Autodesk Inventor part; units mm, degrees
ref_plane "YZ Plane" through (0, 0, 0) normal (1, 0, 0) x (0, 1, 0)
ref_plane "XZ Plane" through (0, 0, 0) normal (0, 1, 0) x (-1, 0, 0)
ref_plane "XY Plane" through (0, 0, 0) normal (0, 0, 1) x (1, 0, 0)
sketch "Sketch1" plane through (0, 0, 0) normal (0, 0, 1) x (1, 0, 0)
  line L0 (-25, -25) -> (25, -25)
  line L1 (25, -25) -> (25, 25)
  line L2 (25, 25) -> (-25, 25)
  line L3 (-25, 25) -> (-25, -25)
  line L4 (-25, -25) -> (25, 25) construction
  line L5 (25, -25) -> (-25, 25) construction
  line L6 (-25, 0) -> (25, 0) construction
  circle A0 centre (-12, 0) radius 1.75
  line L7 (0, 25) -> (0, -25) construction
  circle A1 centre (12, 0) radius 1.75
  line L8 (-25, 25) -> (25, 25)
  line L9 (25, 25) -> (25, 50)
  line L10 (25, 50) -> (-25, 50)
  line L11 (-25, 50) -> (-25, 25)
  line L12 (-20, 45) -> (-17, 45)
  line L13 (-17, 45) -> (-17, 39)
  line L14 (-17, 39) -> (-20, 39)
  line L15 (-20, 39) -> (-20, 45)
  line L16 (20, 45) -> (17, 45)
  line L17 (17, 45) -> (17, 39)
  line L18 (17, 39) -> (20, 39)
  line L19 (20, 39) -> (20, 45)
  point P0 (0, 0)
  dimension "d0" = 50
  dimension "d1" = 50
  dimension "d14" = 3.5
  dimension "d15" = 24
  dimension "d16" = 25
  dimension "d17" = 5
  dimension "d18" = 6
  dimension "d19" = 3
  dimension "d20" = 17
extrude "Extrusion1" add sketch "Sketch1" along normal blind 5
sketch "Sketch2" plane through (-25, -25, 0) normal (0, -1, 0) x (1, 0, 0)
  line L0 (0, 0) -> (50, 0)
  line L1 (0, 5) -> (50, 5)
  line L2 (0, 0) -> (0, 5)
  arc A0 (17.3396, 24.4279) -> (32.6604, 24.4279) centre (25, 18) ccw
  circle A1 centre (25, 18) radius 17 construction
  line L3 (25, 18) -> (25, 0) construction
  line L4 (0, 5) -> (0, 18)
  arc A2 (50, 18) -> (0, 18) centre (25, 18) ccw
  line L5 (50, 18) -> (50, 5)
  line L6 (25, 18) -> (25, 43) construction
  line L7 (17.3396, 24.4279) -> (20.3369, 28)
  line L8 (25, 33.5572) -> (29.6631, 28)
  line L9 (50, 0) -> (50, 5)
  line L10 (20.3369, 28) -> (29.6631, 28)
  arc A3 (32.6604, 24.4279) -> (25, 28) centre (25, 18) ccw
  arc A4 (25, 28) -> (17.3396, 24.4279) centre (25, 18) ccw
  arc A5 (25, 28) -> (17.3396, 24.4279) centre (25, 18) ccw
  arc A6 (32.6604, 24.4279) -> (25, 28) centre (25, 18) ccw
  line L11 (29.6631, 28) -> (32.6604, 24.4279)
  line L12 (20.3369, 28) -> (25, 33.5572)
  dimension "d4" = 20
  dimension "d5" = 34
  dimension "d6" = 18
  dimension "d24" = 80
extrude "Extrusion2" add sketch "Sketch2" against normal blind 8 contours L4 A2 L5 L1 | A4 A3 A0 | L7 L10 A4 | A3 L10 L11 | L12 L8 L10
sketch "Sketch3" plane through (0, 0, 0) normal (1, 0, 0) x (0, 1, 0)
  line L0 (-17, 28) -> (-25, 28)
  line L1 (-17, 8) -> (-17, 5)
  line L2 (-17, 5) -> (50, 5)
  line L3 (50, 0) -> (-25, 0)
  line L4 (-25, 0) -> (-25, 8)
  line L5 (-25, 43) -> (-17, 43)
  line L6 (-17, 43) -> (-17, 28)
  line L7 (-25, 8) -> (-17, 8)
  line L8 (-25, 28) -> (-25, 43)
  line L9 (-25, 8) -> (-25, 28)
  line L10 (-25, 18) -> (31, 18)
  line L11 (9, 29) -> (31, 35)
  line L12 (31, 18) -> (31, 35)
  line L13 (50, 5) -> (50, 0)
  line L14 (9, 29) -> (-17, 28)
  line L15 (31, 18) -> (56.5287, 18)
  line L16 (56.5287, 18) -> (56.5287, 35)
  line L17 (56.5287, 35) -> (31, 35)
  line L18 (31, 35) -> (31, 18)
  point P0 (0, 0)
  dimension "d9" = 26
  dimension "d10" = 22
  dimension "d11" = 11
  dimension "d12" = 17
revolve "Revolution1" cut sketch "Sketch3" angle 360 about axis through (0, -25, 18) along (0, 1, 0) contours L14 L11 L12 L10 L9 L0 | L17 L16 L15 L12
sketch "Sketch4" plane through (-25, -25, 0) normal (-1, 0, 0) x (0, 0, 1)
  line L0 (5, 8) -> (18, 8)
  line L1 (5, 75) -> (5, 8)
  line L2 (18, 8) -> (5, 58)
  point P0 (0, 25)
  dimension "d21" = 50
extrude "Extrusion3" add sketch "Sketch4" against normal blind 4
mirror "Mirror1" about plane through (0, 0, 0) normal (1, 0, 0) of "Extrusion3"
sketch "Szkic5" plane through (-25, -25, 0) normal (0, -1, 0) x (1, 0, 0)
  circle A0 centre (25, 18) radius 10
  line L0 (20.3369, 28) -> (29.6631, 28)
  line L1 (17.3396, 24.4279) -> (20.3369, 28)
  line L2 (29.6631, 28) -> (32.6604, 24.4279)
  point P0 (25, 0)
extrude "Wyciągnięcie proste4" cut sketch "Szkic5" against normal up to next contours A0 L0 L2 | L1 L0 A0
properties part number "proxxon_mount"
Build history of the part. All positions in model axes, mm. A direction names the side the tool comes from. Give positions to 0.01 mm unless a question says otherwise; leave off trailing zeros. Loops run counter-clockwise (first coordinate to the right, second up) from the corner with the lowest first, then second, coordinate; pieces in that order, holes last. Notation, with made-up numbers: (6.5, 40) - (55.5, 40) arc R26 ccw to (55.5, 70) - close; hole circle Ø6 at (60, 66). An arc over 180 degrees is marked (long way). Use a Markdown table: item, result.
(1) Band-saw the part on C-C (z = 9.5). Give the cut face in (x, y).
Taken from the geometry:
| item | result |
|---|---|
| outline | (-25, -25) - (-5.27, -25) - (-5.27, -17) - (-21, -17) - (-21, 15.69) - (-25, 15.69) - close; (5.27, -25) - (25, -25) - (25, 15.69) - (21, 15.69) - (21, -17) - (5.27, -17) - close |
(2) Drop flat-ended pins along their axis: pin 1 Ø12 at (x, z) = (0, 18) entering from +Y; pin 2 Ø3 at (x, y) = (2, 7) entering from +Z; pin 3 Ø3 at (x, y) = (-4.5, 41.5) entering from +Z. Give the stop position or say it passes through.
Taken from the geometry:
| item | result |
|---|---|
| pin 1 | through |
| pin 2 | z = 5 |
| pin 3 | z = 2.09 |
(3) Band-saw the part on A-A (x = 0). Give the cut face in (y, z).
Taken from the geometry:
| item | result |
|---|---|
| outline | (-25, 0) - (50, 0) - (50, 1) - (31, 1) - (16.33, 5) - (-17, 5) - (-17, 8) - (-25, 8) - close; (-25, 28) - (-17, 28) - (-17, 43) - (-25, 43) - close |
(4) Wall check: line 1 along Y through (x, z) = (-12, 1.25); line 2 along Z through (x, y) = (0, -19.75); line 3 along X through (y, z) = (17.5, 8.5). Give the ranges that are in metal, low to high.
Taken from the geometry:
| item | result |
|---|---|
| line 1 | -25 to -1.75, 1.75 to 50 |
| line 2 | 0 to 8, 28 to 43 |
| line 3 | -25 to -21, 21 to 25 |
(5) Which spindle directions (+Z, -Z, +X, -X, +Y, -Y) get a long thin tool onto all of the face, cutting with end or side? Do faces 1 (the face through (-21, -3, 9)), 2 (the face through (17, 42, 2)), 3 (the face through (0, -21, 28)). Say none if no direction does.
Taken from the geometry:
| item | result |
|---|---|
| face 1 | +Z, +Y |
| face 2 | +Z, -Z |
| face 3 | +Y, -Y |
(6) Band-saw the part on D-D (x = 12). Give the cut face in (y, z), and give its area (3 significant figures).
Taken from the geometry:
| item | result |
|---|---|
| outline | (-25, 0) - (-1.75, 0) - (-1.75, 5) - (-17, 5) - (-17, 39.93) - (-25, 39.93) - close; (1.75, 0) - (50, 0) - (50, 5) - (1.75, 5) - close |
| area | 637 mm2 |
(7) Pull direction X, two halves, no side cores. Call faces 4 (the face through (6.14, -21.06, 26.24)), 5 (the face through (-25, 5, 7)), 6 (the face through (23.03, 8.35, 11.41)): +X half, -X half, draft (parallel to the pull), parting line (faces both ways), or undercut.
Taken from the geometry:
| item | result |
|---|---|
| face 4 | undercut |
| face 5 | -X half |
| face 6 | draft |
(8) Band-saw the part on B-B (y = 0). Give the cut face in (x, z).
Taken from the geometry:
| item | result |
|---|---|
| outline | (-25, 0) - (-13.75, 0) - (-13.75, 5) - (-21, 5) - (-21, 13.58) - (-25, 13.58) - close; (-10.25, 0) - (10.25, 0) - (10.25, 5) - (-10.25, 5) - close; (13.75, 0) - (25, 0) - (25, 13.58) - (21, 13.58) - (21, 5) - (13.75, 5) - close |
